Could you check a few things on this model? Use its own coordinates, in mm. A direction names the side the tool comes from. Round coordinates to 2 decimals unless told otherwise and drop trailing zeros. Loops run counter-clockwise (first coordinate to the right, second up) from the corner with the lowest first, then second, coordinate; pieces in that order, holes last. Notation, with made-up numbers: (39, 65) -> (72, 65) arc R21 ccw to (72, 85) -> close; hole circle Ø1 at (-26.5, 56). An arc over 180 degrees is marked (long way). One line per item, written item: value.
```python
from build123d import *

# Parameters (mm, degrees)
BOSS_EXTRUDE1_DEPTH = 19.05
SKETCH2_R           = 1.651
CUT_EXTRUDE1_DEPTH  = 12.7
FILLET1_R           = 0.254


with BuildPart() as part:
    # Sketch1 → Boss-Extrude1 (new body)
    with BuildSketch(Plane(origin=(0, 0, 0), x_dir=(1, 0, 0), z_dir=(0, 1, 0))):
        with BuildLine():
            Line((2.54, -0.635), (3.110851973, -0.635))
            ThreePointArc((3.110851973, -0.635), (0, -3.175), (-3.110851973, -0.635))
            Line((-3.110851973, -0.635), (-2.54, -0.635))
            Line((-2.54, -0.635), (-2.54, 0.635))
            Line((-2.54, 0.635), (-3.110851973, 0.635))
            ThreePointArc((-3.110851973, 0.635), (0, 3.175), (3.110851973, 0.635))
            Line((3.110851973, 0.635), (2.54, 0.635))
            Line((2.54, 0.635), (2.54, -0.635))
        make_face()
    extrude(amount=BOSS_EXTRUDE1_DEPTH)

    # Sketch2 → Cut-Extrude1 (cut)
    with BuildSketch(Plane(origin=(0, 19.05, 0), x_dir=(1, 0, 0), z_dir=(0, 1, 0))):
        Circle(SKETCH2_R)
    extrude(amount=-CUT_EXTRUDE1_DEPTH, mode=Mode.SUBTRACT)

    # Fillet1
    fillet1_edges = [part.edges().sort_by_distance(p)[0] for p in [
        (2.54, 9.525, 0.635),
        (-2.54, 9.525, 0.635),
        (-2.54, 9.525, -0.635),
        (2.54, 9.525, -0.635),
    ]]
    fillet(fillet1_edges, radius=FILLET1_R)


solid = part.part
```
Item 1: I need wall thicknesses on line 1 (X direction, y = 7.25, z = 0); line 2 (Y direction, x = -1.25, z = -0.75); line 3 (Z direction, x = 2.75, y = 16.5). Which ranges of each line are inside material? Lowest first, please. Write a range as from..to.
Output:
line 1: x = -2.54..-1.65, 1.65..2.54
line 2: y = 0..6.35
line 3: z = -1.59..-0.63, 0.63..1.59
Item 2: Will these pins go through, and if not, where does the flat tip stop? pin 1 Ø1.5 at (y, z) = (10.5, -2) entering from +X; pin 2 Ø2 at (x, y) = (2.5, 11.5) entering from +Z; pin 3 Ø2 at (x, y) = (-1.5, 6) entering from -Z.
Output:
pin 1: stops at x = 2.92
pin 2: stops at z = 2.8
pin 3: stops at z = -3.14
Item 3: If we section it at C-C on z = 0: List the corners of the cut face in (x, y) for me, plus the area to 3 significant figures.
Output:
outline: (-2.54, 0) -> (2.54, 0) -> (2.54, 19.05) -> (1.65, 19.05) -> (1.65, 6.35) -> (-1.65, 6.35) -> (-1.65, 19.05) -> (-2.54, 19.05) -> close
area: 54.8 mm²
Item 4: If we mould it in two halves opening along X, with no side actions, what happens to faces 3 (the face through (-1.3, 19.05, 1.4)), 4 (the face through (0, 6.35, 0)), 5 (the face through (0.061, 9.392, 3.174))? For each: released by +X, released by -X, zero draft, split by the parting line, or undercut.
Output:
face 3: zero draft
face 4: undercut
face 5: split by the parting line
Item 5: If we section it at A-A on x = 0: List the corners of the cut face in (y, z) for me (3 decimals).
Output:
outline: (0, -3.175) -> (19.05, -3.175) -> (19.05, -1.651) -> (6.35, -1.651) -> (6.35, 1.651) -> (19.05, 1.651) -> (19.05, 3.175) -> (0, 3.175) -> close
Item 6: If we section it at D-D on y = 2.5: List the corners of the cut face in (x, z) for me (3 decimals).
Output:
outline: (-3.111, -0.635) arc R3.175 ccw to (3.111, -0.635) -> (2.794, -0.635) arc R0.254 cw to (2.54, -0.381) -> (2.54, 0.381) arc R0.254 cw to (2.794, 0.635) -> (3.111, 0.635) arc R3.175 ccw to (-3.111, 0.635) -> (-2.794, 0.635) arc R0.254 cw to (-2.54, 0.381) -> (-2.54, -0.381) arc R0.254 cw to (-2.794, -0.635) -> close
Item 7: If we section it at B-B on y = 15: List the corners of the cut face in (x, z) for me (3 decimals), plus the area to 3 significant figures.
Output:
outline: (-3.111, -0.635) arc R3.175 ccw to (3.111, -0.635) -> (2.794, -0.635) arc R0.254 cw to (2.54, -0.381) -> (2.54, 0.381) arc R0.254 cw to (2.794, 0.635) -> (3.111, 0.635) arc R3.175 ccw to (-3.111, 0.635) -> (-2.794, 0.635) arc R0.254 cw to (-2.54, 0.381) -> (-2.54, -0.381) arc R0.254 cw to (-2.794, -0.635) -> close; hole circle Ø3.302 at (0, 0)
area: 21.6 mm²
Item 8: For faces 1 (the face through (0, 0, 0)), 2 (the face through (1.525, 12.789, 0.632)), which set-ups out of +Z, -Z, +X, -X, +Y, -Y let a thin tool reach every point of the face, with its end or its side?
Output:
face 1: +Z, -Z, +X, -X, -Y
face 2: +Y
